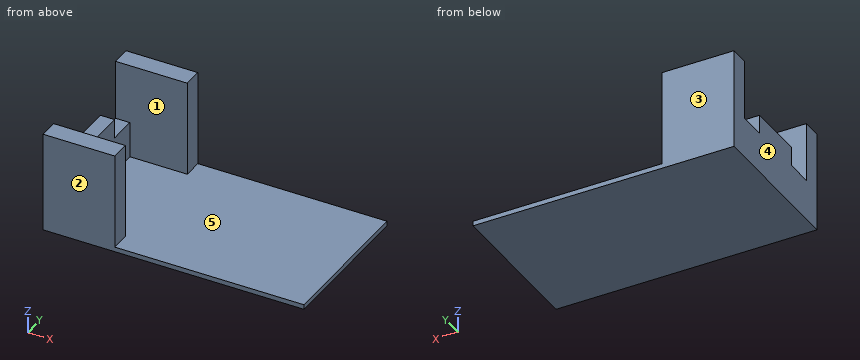
```python
from build123d import *

# Parameters (mm, degrees)
SKETCH_W     = 109
SKETCH_H     = 63
PAD_DEPTH    = 2
SKETCH001_W  = 30
SKETCH001_H  = 8
PAD001_DEPTH = 40
SKETCH002_W  = 6
SKETCH002_H  = 47
PAD002_DEPTH = 15
SKETCH003_W  = 6
SKETCH003_H  = 24
PAD003_DEPTH = 8


with BuildPart() as part:
    # Sketch → Pad (new body)
    with BuildSketch(Plane.XY):
        Rectangle(SKETCH_W, SKETCH_H)
    extrude(amount=PAD_DEPTH)

    # Sketch001 → Pad001 (new body)
    with BuildSketch(Plane.XY.offset(2)):
        with Locations((-39.5, 27.5)):
            Rectangle(SKETCH001_W, SKETCH001_H)
        with Locations((-39.5, -27.5)):
            Rectangle(SKETCH001_W, SKETCH001_H)
    extrude(amount=PAD001_DEPTH)

    # Sketch002 → Pad002 (new body)
    with BuildSketch(Plane.XY.offset(2)):
        with Locations((-51.5, 0)):
            Rectangle(SKETCH002_W, SKETCH002_H)
    extrude(amount=PAD002_DEPTH)

    # Sketch003 → Pad003 (new body)
    with BuildSketch(Plane.XY.offset(17)):
        with Locations((-51.5, 0)):
            Rectangle(SKETCH003_W, SKETCH003_H)
    extrude(amount=PAD003_DEPTH)


solid = part.part
```
Geometry check sheet. Reference: the model listing, model coordinates, mm. Face numbers are marked on the shaded views. A direction names the side the tool comes from. Coordinates: 2 decimals unless noted, no trailing zeros. Loops run counter-clockwise (first coordinate to the right, second up) from the corner with the lowest first, then second, coordinate; pieces in that order, holes last.
Item 1: Sectioned sample at B-B, the plane z = 19. Record the boundary of the cut face in (x, y).
Item 2: Thickness scan on line 1 (Y direction, x = -49, z = 18); line 2 (Z direction, x = -15, y = -11); line 3 (X direction, y = 26.5, z = 22.5). Record the ranges inside material, lowest first.
Item 3: Sectioned sample at D-D, the plane x = -39. Record the boundary of the cut face in (y, z).
Item 4: Release check for a two-part mould opening along Y. For the marked faces 3, 4 and 5 record: released by +Y, released by -Y, zero draft, split by the parting line, or undercut.
Item 5: Access from +Z, -Z, +X, -X, +Y, -Y to the whole of each face (thin tool, end or side, straight path). Record for the marked faces 1 and 2.
Item 6: Sectioned sample at C-C, the plane y = -2.5. Record the boundary of the cut face in (x, z).
Item 7: Sectioned sample at A-A, the plane z = 27.5. Record the boundary of the cut face in (x, y).
Item 8: Go/stop test with flat-tipped pins: pin 1 Ø1.5 at (x, y) = (-13, -22) entering from +Z; pin 2 Ø9 at (y, z) = (27, 18.5) entering from +X; pin 3 Ø2 at (y, z) = (-5, 23.5) entering from +X. Record where each tip stops, or that it passes through.
Check result:
1. outline: (-54.5, -31.5) - (-24.5, -31.5) - (-24.5, -23.5) - (-54.5, -23.5) - close; (-54.5, -12) - (-48.5, -12) - (-48.5, 12) - (-54.5, 12) - close; (-54.5, 23.5) - (-24.5, 23.5) - (-24.5, 31.5) - (-54.5, 31.5) - close
2. line 1: y = -31.5 to -23.5, -12 to 12, 23.5 to 31.5
2. line 2: z = 0 to 2
2. line 3: x = -54.5 to -24.5
3. outline: (-31.5, 0) - (31.5, 0) - (31.5, 42) - (23.5, 42) - (23.5, 2) - (-23.5, 2) - (-23.5, 42) - (-31.5, 42) - close
4. face 3: released by +Y
4. face 4: zero draft
4. face 5: undercut
5. face 1: +Z, +X
5. face 2: +Z, -Z, +X, -X, -Y
6. outline: (-54.5, 0) - (54.5, 0) - (54.5, 2) - (-48.5, 2) - (-48.5, 25) - (-54.5, 25) - close
7. outline: (-54.5, -31.5) - (-24.5, -31.5) - (-24.5, -23.5) - (-54.5, -23.5) - close; (-54.5, 23.5) - (-24.5, 23.5) - (-24.5, 31.5) - (-54.5, 31.5) - close
8. pin 1: stops at z = 2
8. pin 2: stops at x = -24.5
8. pin 3: stops at x = -48.5
